from build123d import *

# Parameters (mm, degrees)
F0_W     = 15
F0_H     = 15
F0_H_2   = 10
F0_W_2   = 5
F0_H_3   = 5
F1_DEPTH = 15
F2_R     = 1.4
F3_DEPTH = 25
F2_R_2   = 3.5
F4_DEPTH = 8
F5_R     = 3.5
F5_R_2   = 1.45
F6_DEPTH = 8
F7_DEPTH = 25


with BuildPart() as f1:
    # F0 (on Top) → F1 (new body)
    with BuildSketch(Plane.XY):
        Polygon((0, 15), (0, 0), (15, 8), (15, 23.125), align=None)
        Polygon((0, 65), (0, 15), (15, 23.125), (15, 65), align=None)
        Polygon((15, 23.125), (15, 8), (121.875, 65), (92.3076923077, 65), align=None)
        Polygon((15, 8), (0, 0), (0, -12.10534852), (15, -12.10534852), align=None)
        Polygon((15, 80), (15, 65), (92.3076923077, 65), (120, 80), align=None)
        with Locations((7.5, 72.5)):
            Rectangle(F0_W, F0_H)
        with Locations((7.5, 85)):
            Rectangle(F0_W, F0_H_2)
        Polygon((92.3076923077, 65), (121.875, 65), (150, 80), (145, 80), (120, 80), align=None)
        Polygon((150, 80), (121.875, 65), (150, 65), align=None)
        with Locations((147.5, 82.5)):
            Rectangle(F0_W_2, F0_H_3)
    extrude(amount=F1_DEPTH)

    # F2 (on face) → F3 (cut)
    with BuildSketch(Plane.YZ.offset(15)):
        with Locations((85, 7.5)):
            Circle(F2_R)
    extrude(amount=-F3_DEPTH, mode=Mode.SUBTRACT)

    # F2 (on face) → F4 (cut)
    with BuildSketch(Plane.YZ.offset(15)):
        with Locations((85, 7.5)):
            Circle(F2_R_2)
        with Locations((85, 7.5)):
            Circle(F2_R, mode=Mode.SUBTRACT)
    extrude(amount=-F4_DEPTH, mode=Mode.SUBTRACT)

    # F5 (on face) → F6 (cut)
    with BuildSketch(Plane.YZ.offset(15)):
        with Locations((-2.05267426, 7.5)):
            Circle(F5_R)
        with Locations((-2.05267426, 7.5)):
            Circle(F5_R_2, mode=Mode.SUBTRACT)
    extrude(amount=-F6_DEPTH, mode=Mode.SUBTRACT)

    # F7 (cut): a face of the model
    f7_faces = [f1.faces().sort_by_distance(p)[0] for p in [
        (15, -2.05267426, 7.5),
    ]]
    extrude(f7_faces, amount=-F7_DEPTH, mode=Mode.SUBTRACT)


solid = f1.part
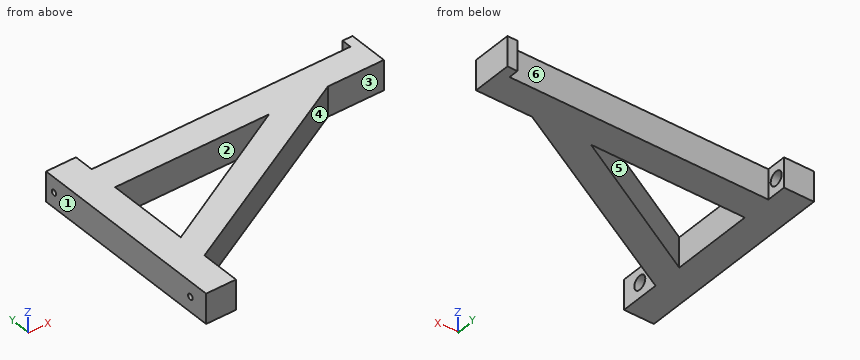
The model under review builds one solid part; all positions refer to its coordinate system, in mm. Face numbers are marked on the shaded views. A direction names the side the tool comes from. Round coordinates to 2 decimals unless told otherwise and drop trailing zeros. Write each loop counter-clockwise with the first axis right and the second up, starting at its lowest first coordinate (ties: lowest second). Pieces come first, ordered by that corner, then holes. Notation, with made-up numbers: M -31,29 L -18,29 A34 cw -18,66 Z; hole C -11,72 d3. An arc over 180 degrees is marked long. Answer as CSV lines item,"result". Start each with the question number.
Q1. Consider section A-A, the plane z = 13.25. Give the boundary of the cut face in (x, y) (3 decimals).
Q2. Consider section B-B, the plane x = 61. Give the boundary of the cut face in (y, z), then the cut area to 3 significant figures.
Q3. Consider section D-D, the plane y = 10. Give the boundary of the cut face in (x, z), then the cut area to 3 significant figures.
Q4. Tool access review of the marked faces 4, 5 and 6: name each direction out of +Z, -Z, +X, -X, +Y, -Y from which nothing blocks a thin tool from reaching the whole face with its end or side.
Q5. Clearance check with flat-ended pins moving along their axes: P1, Ø7.5, axis at y = -2.5, z = 7.5, coming from the +X side; P2, Ø3, axis at y = 26, z = 9, coming from the +X side; P3, Ø5.5, axis at x = 147.5, z = 8.5, coming from the +Y side. State where each tip first meets the part, or that it passes through.
Q6. The part is to be moulded in two halves that separate along Y. For the marked faces 1, 2 and 3, say which applies: +Y half, -Y half, draft (parallel to the pull), parting line (faces both ways), or undercut.
Q7. Consider section C-C, the plane y = 27.5. Give the boundary of the cut face in (x, z).
Q8. Wall thickness on line 1 along Z through (x, y) = (9.5, 85); line 2 along X through (y, z) = (54, 10.5); line 3 along Y through (x, z) = (11, 6.75): over which ranges is each line inside the solid? List them lowest first.
Result set:
1,outline,"M 0,-12.105 L 15,-12.105 L 15,8 L 121.875,65 L 150,65 L 150,85 L 145,85 L 145,80 L 15,80 L 15,90 L 0,90 Z; hole M 15,23.125 L 92.308,65 L 15,65 Z"
2,outline,"M 32.53,0 L 48.04,0 L 48.04,15 L 32.53,15 Z; M 65,0 L 80,0 L 80,15 L 65,15 Z"
2,area,"458 mm²"
3,outline,"M 0,0 L 18.75,0 L 18.75,15 L 0,15 Z"
3,area,"281 mm²"
4,face 4,"+Z, -Z, +X, -Y"
4,face 5,"+Z, -Z"
4,face 6,"+Z, -Z, +Y"
5,P1,"stops at x = 15"
5,P2,"stops at x = 51.56"
5,P3,"stops at y = 85"
6,face 1,"draft"
6,face 2,"undercut"
6,face 3,"-Y half"
7,outline,"M 0,0 L 15,0 L 15,15 L 0,15 Z; M 23.08,0 L 51.56,0 L 51.56,15 L 23.08,15 Z"
8,line 1,"z = 0 to 4, 11 to 15"
8,line 2,"x = 0 to 15, 72 to 101.25"
8,line 3,"y = -12.11 to -5.47, 1.37 to 81.58, 88.42 to 90"
